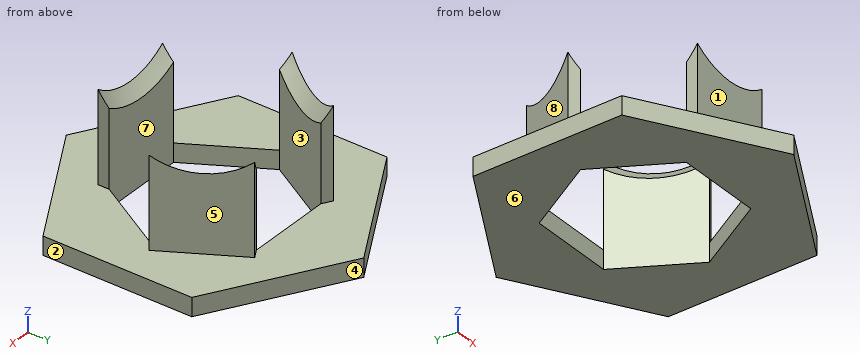
from build123d import *

# Parameters (mm, degrees)
F1_DEPTH = 5
F2_W     = 23.09401
F2_H     = 3
F3_DEPTH = 40


with BuildPart() as f1:
    # F0 (on Top) → F1 (new body)
    with BuildSketch(Plane.XY):
        Polygon((35, -20.207259), (35, 20.207259), (0, 40.414519), (-35, 20.207259), (-35, -20.207259), (0, -40.414519), align=None)
        Polygon((-23.094011, 0), (-11.547005, 20), (11.547005, 20), (23.094011, 0), (11.547005, -20), (-11.547005, -20), align=None, mode=Mode.SUBTRACT)
    extrude(amount=F1_DEPTH)

    # F2 (on face) → F3 (join)
    with BuildSketch(Plane.XY.offset(5)):
        Polygon((-23.094011, 0), (-11.547005, 20), (-14.145082, 21.5), (-25.692087, 1.5), align=None)
        Polygon((14.145082, 21.5), (11.547005, 20), (23.094011, 0), (25.692087, 1.5), align=None)
        with Locations((0, -21.5)):
            Rectangle(F2_W, F2_H)
    extrude(amount=F3_DEPTH)

    # F4 (on face) → F5 (revolve, cut)
    with BuildSketch(Plane.XY.offset(45)):
        with BuildLine():
            Line((0, -30), (0, 30))
            ThreePointArc((0, 30), (-30, 0), (0, -30))
        make_face()
    revolve(axis=Axis((0, 0, 45), (0, -1, 0)), mode=Mode.SUBTRACT)


solid = f1.part
Can you work these out from the model? Positions are in its coordinate system, mm. Face numbers are marked on the shaded views. A direction names the side the tool comes from. Coordinates: 2 decimals unless noted, no trailing zeros. Write each loop counter-clockwise with the first axis right and the second up, starting at its lowest first coordinate (ties: lowest second). Pieces come first, ordered by that corner, then holes. Notation, with made-up numbers: (67, -33.5) -> (117, -33.5) arc R30 ccw to (117, -5.5) -> close; hole circle Ø8 at (47.5, 24.25). An arc over 180 degrees is marked (long way). Write each question's results on one line, items separated by ' | '. Start each with the question number.
Item 1: Please list where these lines run through material, in increasing order: probe 1 along Z at (x, y) = (-1, 25); probe 2 along X at (y, z) = (9, 19); probe 3 along Y at (x, z) = (-10, 13.5).
Item 2: If we section it at B-B, the plane y = -5: Write out the boundary of the cut face in (x, z), and give its area (3 significant figures).
Item 3: I'm going to push flat-ended pins straight in: P1, Ø7, axis at x = 3.5, z = 16.5, coming from the +Y side; P2, Ø2.5, axis at y = -21.5, z = 15, coming from the +X side; P3, Ø3, axis at x = 24.5, z = 7, coming from the +Y side. Where does each tip first touch, or does it pass through?
Item 4: If we section it at C-C, the plane x = -17: Write out the boundary of the cut face in (y, z), and give its area (3 significant figures).
Item 5: On a 3-axis mill with a long thin cutter (end or side, diameter ignored), from which of +Z, -Z, +X, -X, +Y, -Y can I reach the whole of each face in a straight line? I mean the marked faces 5, 6, 7 and 8. Say none if no direction works.
Item 6: If we section it at A-A, the plane z = 12.5: Write out the boundary of the cut face in (x, y), and give its area (3 significant figures).
Item 7: Thinking about a two-plate mould opening in Y: for the marked faces 1, 2, 3 and 4, which applies, released by +Y, released by -Y, zero draft, split by the parting line, or undercut?
Item 8: If we section it at D-D, the plane z = 3.5: Write out the boundary of the cut face in (x, y).
Answer block:
1) probe 1: 0 to 5 | probe 2: -21.36 to -17.9, 17.9 to 21.36 | probe 3: -23 to -20
2) outline: (-35, 0) -> (-20.21, 0) -> (-20.21, 5) -> (-35, 5) -> close; (20.21, 0) -> (35, 0) -> (35, 5) -> (20.21, 5) -> close | area: 148 mm²
3) P1: y = -20 | P2: x = 11.55 | P3: y = 6.16
4) outline: (-30.6, 0) -> (-10.56, 0) -> (-10.56, 5) -> (-30.6, 5) -> close; (10.56, 0) -> (30.6, 0) -> (30.6, 5) -> (16.56, 5) -> (16.56, 26.64) arc R24.72 cw to (10.56, 22.65) -> close | area: 317 mm²
5) face 5: +Z, +X, +Y | face 6: -Z, +X, -X, +Y, -Y | face 7: +Z, -Z | face 8: +Z, -X, +Y
6) outline: (-25.69, 1.5) -> (-23.09, 0) -> (-11.55, 20) -> (-14.15, 21.5) -> close; (-11.55, -23) -> (11.55, -23) -> (11.55, -20) -> (-11.55, -20) -> close; (11.55, 20) -> (23.09, 0) -> (25.69, 1.5) -> (14.15, 21.5) -> close | area: 208 mm²
7) face 1: released by -Y | face 2: zero draft | face 3: undercut | face 4: released by +Y
8) outline: (-35, -20.21) -> (0, -40.41) -> (35, -20.21) -> (35, 20.21) -> (0, 40.41) -> (-35, 20.21) -> close; hole (-23.09, 0) -> (-11.55, -20) -> (11.55, -20) -> (23.09, 0) -> (11.55, 20) -> (-11.55, 20) -> close
